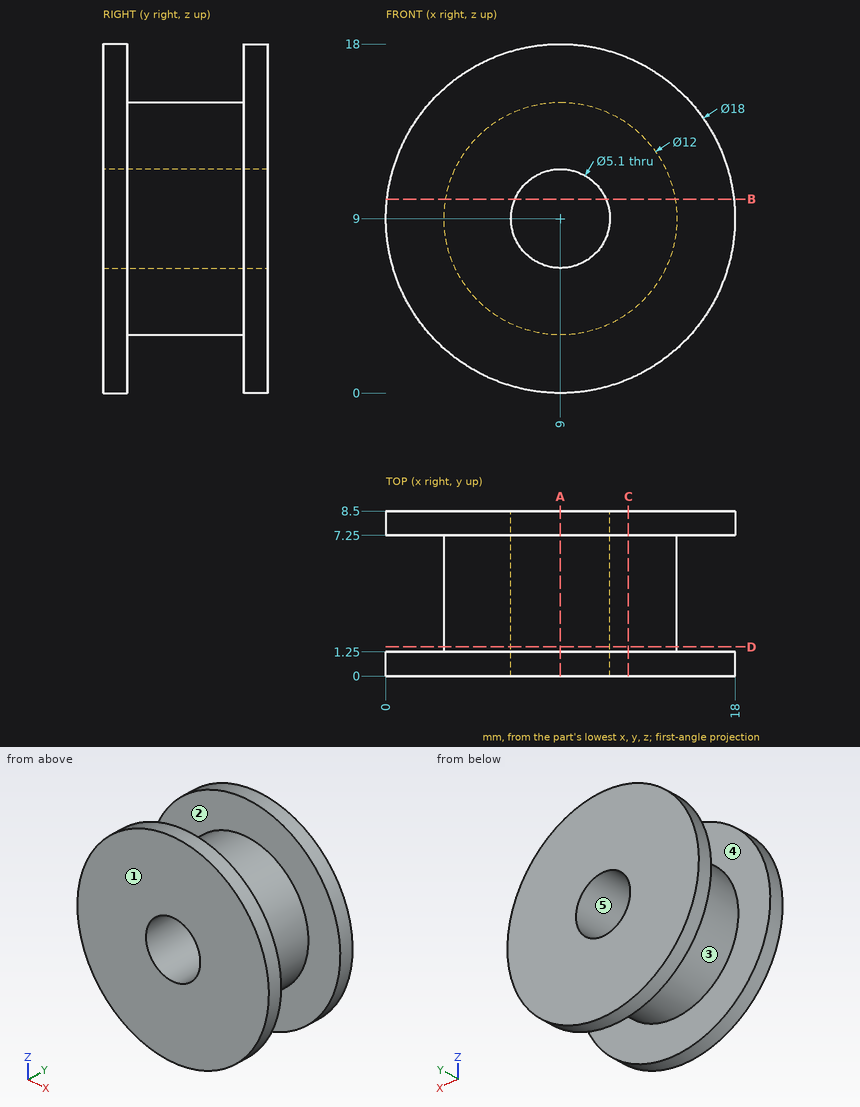
Geometry: see drawing. Coordinates: mm, zero at the bounding-box minimum. A direction names the side the tool comes from. Give positions to 0.01 mm unless a question says otherwise; leave off trailing zeros. Order: outer loops, then holes, each group sorted by start corner. A loop starts at its lowest first (then second) coordinate and runs counter-clockwise, first axis right, second up.
1. Draft query along X for the marked faces 3, 4 and 5. Return one class per face: released by +X, released by -X, zero draft, split by the parting line, or undercut.
Computed:
face 3: split by the parting line
face 4: zero draft
face 5: undercut
2. Set-up query: the marked faces 1 and 2. Return all of +Z, -Z, +X, -X, +Y, -Y with unobstructed straight access to the full face (end or side cutting, diameter ignored); none if empty.
Computed:
face 1: +Z, -Z, +X, -X, -Y
face 2: none
3. Line query: probe 1 along Y at (x, z) = (3.75, 2.5); probe 2 along X at (y, z) = (3.75, 9); probe 3 along Z at (x, y) = (9.5, 8). Output: solid intervals per line, ascending.
Computed:
probe 1: y = 0 to 1.25, 7.25 to 8.5
probe 2: x = 3 to 6.45, 11.55 to 15
probe 3: z = 0.01 to 6.5, 11.5 to 17.99
4. Cut plane C-C (x = 12.5). Return loops of the section in (y, z), and give its area (3 significant figures).
Computed:
outline: (0, 0.71) - (1.25, 0.71) - (1.25, 4.13) - (7.25, 4.13) - (7.25, 0.71) - (8.5, 0.71) - (8.5, 17.29) - (7.25, 17.29) - (7.25, 13.87) - (1.25, 13.87) - (1.25, 17.29) - (0, 17.29) - close
area: 99.9 mm2
5. Pin query (flat end, axial travel): pin 1 Ø4 at (y, z) = (3, 13) entering from -X; pin 2 Ø1.5 at (y, z) = (1, 8.5) entering from +X; pin 3 Ø1 at (x, y) = (5.5, 6) entering from +Z; pin 4 Ø4 at (x, y) = (3, 3) entering from -Z. Return the tip coordinate at first contact, or that it passes through.
Computed:
pin 1: stops at x = 0.53
pin 2: stops at x = 18
pin 3: stops at z = 14.2
pin 4: stops at z = 1.54
6. Cut plane D-D (y = 1.5). Return loops of the section in (x, z).
Computed:
outline: circle Ø12 at (9, 9); hole circle Ø5.1 at (9, 9)
7. Cut plane A-A (x = 9). Return loops of the section in (y, z), and give its area (4 significant figures).
Computed:
outline: (0, 0) - (1.25, 0) - (1.25, 3) - (7.25, 3) - (7.25, 0) - (8.5, 0) - (8.5, 6.45) - (0, 6.45) - close; (0, 11.55) - (8.5, 11.55) - (8.5, 18) - (7.25, 18) - (7.25, 15) - (1.25, 15) - (1.25, 18) - (0, 18) - close
area: 73.65 mm2
8. Cut plane B-B (z = 10). Return loops of the section in (x, y).
Computed:
outline: (0.06, 0) - (6.65, 0) - (6.65, 8.5) - (0.06, 8.5) - (0.06, 7.25) - (3.08, 7.25) - (3.08, 1.25) - (0.06, 1.25) - close; (11.35, 0) - (17.94, 0) - (17.94, 1.25) - (14.92, 1.25) - (14.92, 7.25) - (17.94, 7.25) - (17.94, 8.5) - (11.35, 8.5) - close
